Check sheet for the drawn part. Datum: minimum x, y, z corner. Units: mm. Coordinates: 2 decimals unless noted, no trailing zeros. Answer in a Markdown table with one row per item.
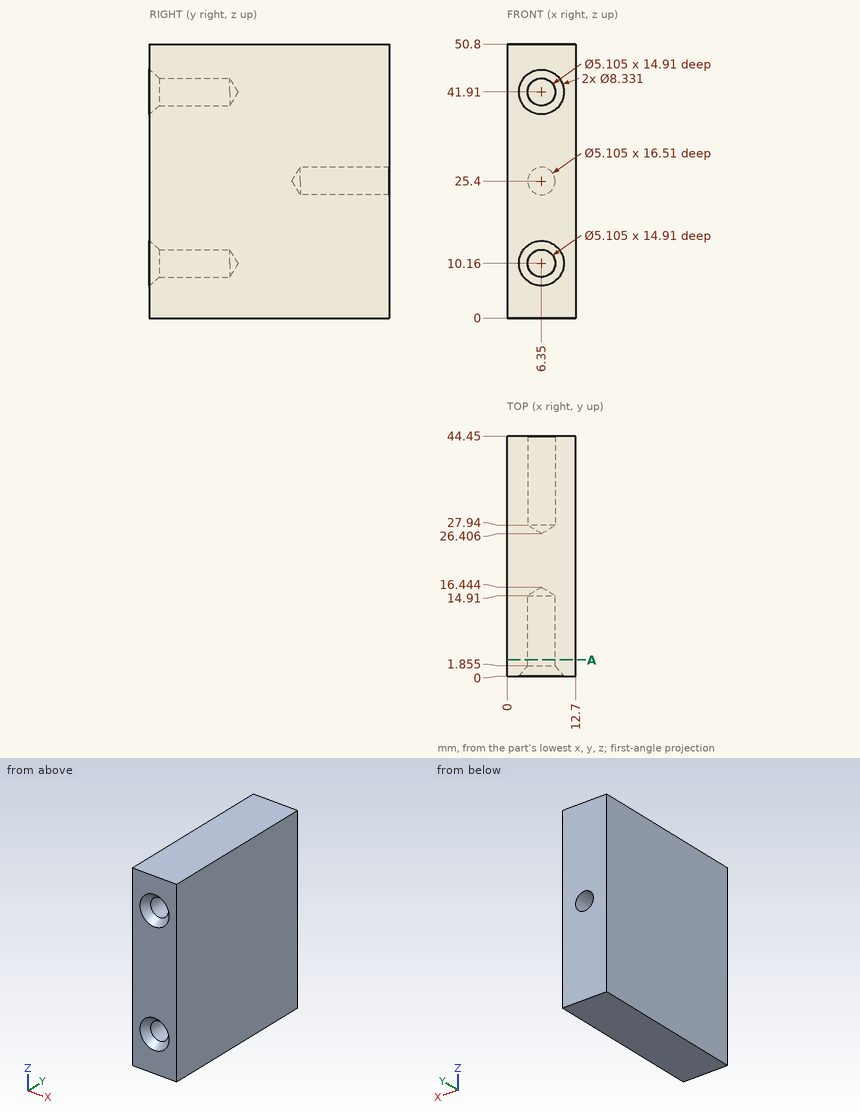
1. Sectioned sample at A-A, the plane y = 3. Count the separate pieces of the cut face and the enclosed holes in it, and give its area (3 significant figures).
Findings below:
| item | result |
|---|---|
| separate pieces | 1 |
| enclosed holes | 2 |
| area | 604 mm² |
2. Go/stop test with a flat-tipped pin: pin 1 (3 mm diameter, centred on y = 13.5, z = 34, fed in from -X). Record where the tip stops, or that it passes through.
Findings below:
| item | result |
|---|---|
| pin 1 | stops at x = 0 |
3. Material ranges on probe 1 along Z at (x, y) = (6.35, 10.5); probe 2 along X at (y, z) = (11.75, 41.91); probe 3 along Z at (x, y) = (6, 12), recorded low to high. Write a range as from..to.
Findings below:
| item | result |
|---|---|
| probe 1 | z = 0..7.61, 12.71..39.36, 44.46..50.8 |
| probe 2 | x = 0..3.8, 8.9..12.7 |
| probe 3 | z = 0..7.63, 12.69..39.38, 44.44..50.8 |
